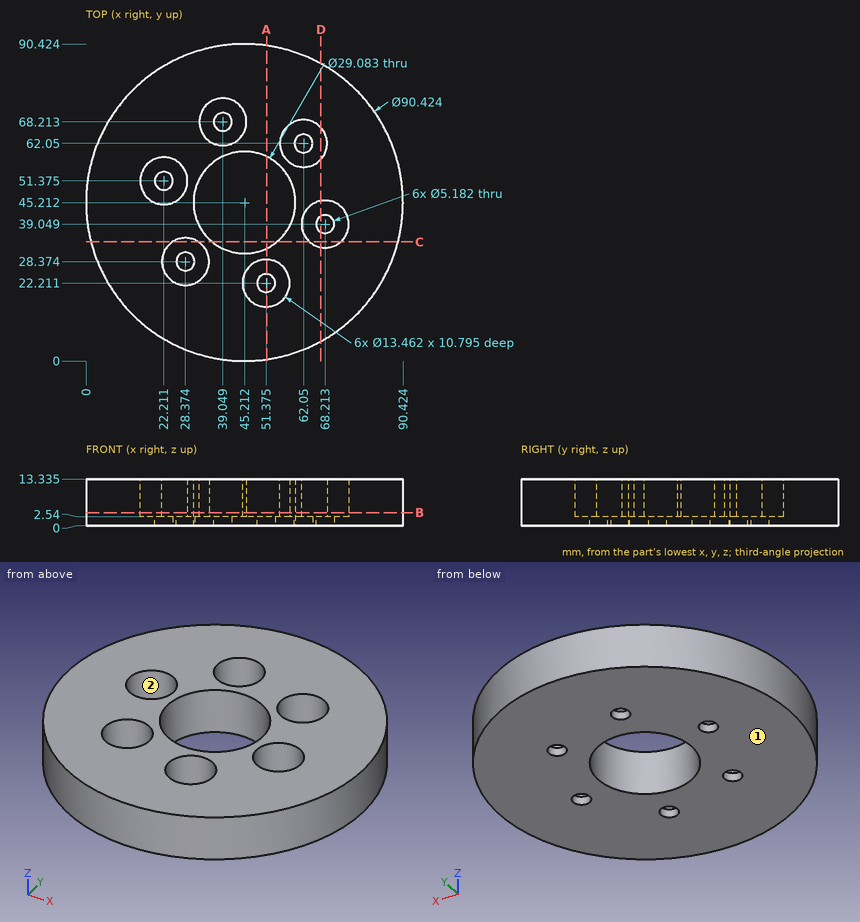
Design review of the part shown in the three views and the two pictorial views. Dimensions are in mm from the part's minimum x, y and z. A direction names the side the tool comes from. Give positions to 0.01 mm unless a question says otherwise; leave off trailing zeros. Write each loop counter-clockwise with the first axis right and the second up, starting at its lowest first coordinate (ties: lowest second). Pieces come first, ordered by that corner, then holes. Notation, with made-up numbers: (9, 13.25) -> (34, 13.25) arc R32 cw to (34, 43.25) -> close; hole circle Ø4 at (82, -7). An arc over 180 degrees is marked (long way). Answer in a Markdown table with one row per item.
1) Add section D-D on x = 67. State the section outline as (y, z) points (1 decimal).
Worked answers:
| item | result |
|---|---|
| outline | (5.6, 0) -> (36.8, 0) -> (36.8, 2.5) -> (32.4, 2.5) -> (32.4, 13.3) -> (5.6, 13.3) -> close; (41.3, 0) -> (84.8, 0) -> (84.8, 13.3) -> (66.6, 13.3) -> (66.6, 2.5) -> (57.5, 2.5) -> (57.5, 13.3) -> (45.7, 13.3) -> (45.7, 2.5) -> (41.3, 2.5) -> close |
2) For L1, parallel to Y at x = 38, z = 6.5 (1 decimal); L2, parallel to X at y = 53, z = 8.75 (1 decimal); L3, parallel to Y at x = 54, z = 5 (1 decimal), list the stretches that pass through material, from the lowest coordinate up. Write a range as [from, to].
Worked answers:
| item | result |
|---|---|
| L1 | [0.6, 32.6], [57.8, 61.6], [74.9, 89.8] |
| L2 | [0.7, 15.7], [28.7, 32.9], [57.5, 89.7] |
| L3 | [0.9, 16], [28.4, 33.6], [56.8, 89.6] |
3) Clearance check with flat-ended pins moving along their axes: P1, Ø4, axis at x = 26, y = 26, coming from the +Z side; P2, Ø3, axis at x = 39.05, y = 68.21, coming from the -Z side; P3, Ø1, axis at y = 43, z = 3.5, coming from the +X side; P4, Ø4, axis at y = 75, z = 3.5, coming from the -X side. State where each tip first meets the part, or that it passes through.
Worked answers:
| item | result |
|---|---|
| P1 | z = 2.54 |
| P2 | through |
| P3 | x = 90.39 |
| P4 | x = 9.55 |
4) Add section B-B on z = 3.75. Count the separate pieces of the cut face and the enclosed holes in it, plus the area to 3 significant figures.
Worked answers:
| item | result |
|---|---|
| separate pieces | 1 |
| enclosed holes | 7 |
| area | 4,900 mm² |
5) Tool access review of the marked faces 1 and 2: name each direction out of +Z, -Z, +X, -X, +Y, -Y from which nothing blocks a thin tool from reaching the whole face with its end or side.
Worked answers:
| item | result |
|---|---|
| face 1 | -Z, +X, -X, +Y, -Y |
| face 2 | +Z |
6) Add section A-A on x = 51.5. State the section outline as (y, z) points (1 decimal), plus the area to 3 significant figures.
Worked answers:
| item | result |
|---|---|
| outline | (0.4, 0) -> (19.6, 0) -> (19.6, 2.5) -> (15.5, 2.5) -> (15.5, 13.3) -> (0.4, 13.3) -> close; (24.8, 0) -> (32.1, 0) -> (32.1, 13.3) -> (28.9, 13.3) -> (28.9, 2.5) -> (24.8, 2.5) -> close; (58.3, 0) -> (90, 0) -> (90, 13.3) -> (58.3, 13.3) -> close |
| area | 686 mm² |
7) Add section C-C on y = 34. State the section outline as (x, z) points (1 decimal), plus the area to 3 significant figures.
Worked answers:
| item | result |
|---|---|
| outline | (1.4, 0) -> (36, 0) -> (36, 13.3) -> (32.1, 13.3) -> (32.1, 2.5) -> (24.7, 2.5) -> (24.7, 13.3) -> (1.4, 13.3) -> close; (54.5, 0) -> (89, 0) -> (89, 13.3) -> (72.7, 13.3) -> (72.7, 2.5) -> (63.8, 2.5) -> (63.8, 13.3) -> (54.5, 13.3) -> close |
| area | 745 mm² |
